Build history of the part. All positions in model axes, mm. Give positions to 0.01 mm unless a question says otherwise; leave off trailing zeros. Order: outer loops, then holes, each group sorted by start corner. A loop starts at its lowest first (then second) coordinate and runs counter-clockwise, first axis right, second up. Notation, with made-up numbers: (1, -10.75) -> (58, -10.75) arc R16 ccw to (58, -5.75) -> close; hole circle Ø11 at (63.5, 71). An arc over 180 degrees is marked (long way). One line per question, with ' | ' between items. Start each with the question number.
(1) Cut at B-B (z = -4.5). Give the cut face in (x, y), then the cut area to 3 significant figures.
(2) Cut at A-A (x = -24). Give the cut face in (y, z).
(3) Drill centre lines: L1, parallel to Z at x = -2.5, y = -0.25; L2, parallel to Z at x = -4.5, y = 4.25; L3, parallel to Y at x = -23.5, z = 2.5. Where is each one in solid material? Low to high. Write a range as from..to.
(4) Pin check, flat tips, straight feed: pin 1 Ø10 at (x, z) = (-5.5, -5.5) entering from -Y; pin 2 Ø1 at (x, y) = (-27.5, 4.5) entering from -Z; pin 3 Ø2 at (x, y) = (-23, 4.5) entering from +Z. Stop position of each tip, or through.
(5) Cut at C-C (y = -6). Give the cut face in (x, z), then the cut area to 3 significant figures.
from build123d import *

# Parameters (mm, degrees)
SKETCH1_R           = 8.5
BOSS_EXTRUDE1_DEPTH = 31
SKETCH1_2_R         = 8.5
BOSS_EXTRUDE2_DEPTH = 2
SKETCH2_R           = 8.5
BOSS_EXTRUDE3_DEPTH = 2


with BuildPart() as part:
    # Sketch1 → Boss-Extrude1 (new body)
    with BuildSketch(Plane(origin=(0, 0, 0), x_dir=(0, 0, -1), z_dir=(1, 0, 0))):
        Circle(SKETCH1_R)
    extrude(amount=-BOSS_EXTRUDE1_DEPTH)

    # Sketch1<2> → Boss-Extrude2 (add)
    with BuildSketch(Plane(origin=(0, 0, 0), x_dir=(0, 0, -1), z_dir=(1, 0, 0))):
        Circle(SKETCH1_2_R)
    extrude(amount=BOSS_EXTRUDE2_DEPTH)

    # Sketch2 → Boss-Extrude3 (add)
    with BuildSketch(Plane.ZY.offset(31)):
        Circle(SKETCH2_R)
    extrude(amount=BOSS_EXTRUDE3_DEPTH)


solid = part.part
Result set:
1) outline: (-33, -7.21) -> (2, -7.21) -> (2, 7.21) -> (-33, 7.21) -> close | area: 505 mm2
2) outline: circle Ø17 at (0, 0)
3) L1: z = -8.5..8.5 | L2: z = -7.36..7.36 | L3: y = -8.12..8.12
4) pin 1: stops at y = -8.49 | pin 2: stops at z = -7.5 | pin 3: stops at z = 7.75
5) outline: (-33, -6.02) -> (2, -6.02) -> (2, 6.02) -> (-33, 6.02) -> close | area: 421 mm2
